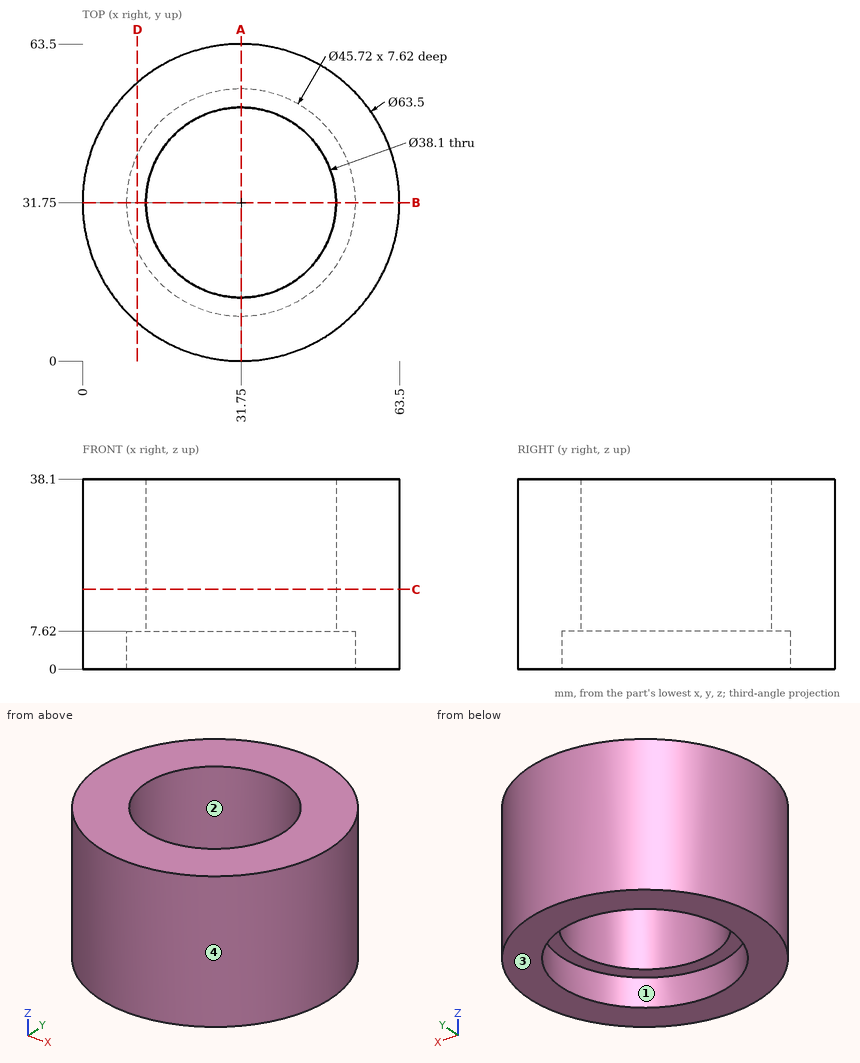
Design review of the part shown in the three views and the two pictorial views. Dimensions are in mm from the part's minimum x, y and z. Coordinates: 2 decimals unless noted, no trailing zeros. Order: outer loops, then holes, each group sorted by start corner. A loop starts at its lowest first (then second) coordinate and runs counter-clockwise, first axis right, second up. Notation, with made-up numbers: (86, 66.25) - (102, 66.25) arc R12 ccw to (102, 77.25) - close; hole circle Ø3 at (75.25, -28.5). An arc over 180 degrees is marked (long way). One line per question, with ' | ' between items.
Q1. Consider section C-C, the plane z = 16. Give the boundary of the cut face in (x, y), then the cut area to 3 significant figures.
Answer key:
outline: circle Ø63.5 at (31.75, 31.75); hole circle Ø38.1 at (31.75, 31.75) | area: 2,030 mm2
Q2. Consider section A-A, the plane x = 31.75. Give the boundary of the cut face in (y, z), then the cut area to 3 significant figures.
Answer key:
outline: (0, 0) - (8.89, 0) - (8.89, 7.62) - (12.7, 7.62) - (12.7, 38.1) - (0, 38.1) - close; (50.8, 7.62) - (54.61, 7.62) - (54.61, 0) - (63.5, 0) - (63.5, 38.1) - (50.8, 38.1) - close | area: 910 mm2
Q3. To check wall thickness, follow line 1 along X through (y, z) = (31, 20); line 2 along Y through (x, z) = (31.75, 21); line 3 along Y through (x, z) = (31.75, 4.25). State the ranges of each line that lie inside material, in increasing order.
Answer key:
line 1: x = 0.01 to 12.71, 50.79 to 63.49 | line 2: y = 0 to 12.7, 50.8 to 63.5 | line 3: y = 0 to 8.89, 54.61 to 63.5
Q4. Clearance check with flat-ended pins moving along their axes: pin 1 Ø4 at (x, y) = (18, 11.5) entering from -Z; pin 2 Ø5 at (y, z) = (7.5, 19.5) entering from +X; pin 3 Ø5 at (x, z) = (49, 16.5) entering from +Y; pin 4 Ø5 at (x, z) = (48.5, 24.5) entering from -Y. State where each tip first meets the part, or that it passes through.
Answer key:
pin 1: stops at z = 0 | pin 2: stops at x = 54.88 | pin 3: stops at y = 59.87 | pin 4: stops at y = 3.38
Q5. The part is to be moulded in two halves that separate along Y. For the marked faces 1, 2, 3 and 4, say which applies: +Y half, -Y half, draft (parallel to the pull), parting line (faces both ways), or undercut.
Answer key:
face 1: undercut | face 2: undercut | face 3: draft | face 4: parting line
Q6. Consider section D-D, the plane x = 11. Give the boundary of the cut face in (y, z).
Answer key:
outline: (7.72, 0) - (22.16, 0) - (22.16, 7.62) - (41.34, 7.62) - (41.34, 0) - (55.78, 0) - (55.78, 38.1) - (7.72, 38.1) - close
